from build123d import *

# Parameters (mm, degrees)
SKETCH1_W           = 10
SKETCH1_H           = 2.7
BOSS_EXTRUDE1_DEPTH = 2.7


with BuildPart() as part:
    # Sketch1 → Boss-Extrude1 (new body)
    with BuildSketch(Plane(origin=(0, 0, 0), x_dir=(0, 0, -1), z_dir=(1, 0, 0))):
        with BuildLine():
            Line((-100, -44), (-100, -60))
            Line((-100, -60), (-80, -60))
            Line((-80, -60), (-80, -50))
            Line((-80, -50), (80, -50))
            Line((80, -50), (80, -60))
            Line((80, -60), (100, -60))
            Line((100, -60), (100, -44))
            Line((100, -44), (97.3, -44))
            Line((97.3, -44), (97.3, -34))
            Line((97.3, -34), (100, -34))
            Line((100, -34), (100, -24))
            Line((100, -24), (97.3, -24))
            Line((97.3, -24), (97.3, -14))
            Line((97.3, -14), (100, -14))
            Line((100, -14), (100, -4))
            Line((100, -4), (97.3, -4))
            Line((97.3, -4), (97.3, 6))
            Line((97.3, 6), (100, 6))
            Line((100, 6), (100, 16))
            Line((100, 16), (97.3, 16))
            Line((97.3, 16), (97.3, 26))
            Line((97.3, 26), (100, 26))
            Line((100, 26), (100, 36))
            Line((100, 36), (97.3, 36))
            Line((97.3, 36), (97.3, 46))
            Line((97.3, 46), (100, 46))
            Line((100, 46), (100, 60))
            Line((100, 60), (75.851854343, 53.529523872))
            Line((75.851854343, 53.529523872), (76.550665765, 50.921524141))
            Line((76.550665765, 50.921524141), (66.891407502, 48.33333369))
            Line((66.891407502, 48.33333369), (66.19259608, 50.941333421))
            Line((66.19259608, 50.941333421), (56.533337817, 48.35314297))
            Line((56.533337817, 48.35314297), (57.232149239, 45.745143239))
            Line((57.232149239, 45.745143239), (47.572890976, 43.156952788))
            Line((47.572890976, 43.156952788), (46.874079554, 45.764952519))
            Line((46.874079554, 45.764952519), (37.214821291, 43.176762068))
            Line((37.214821291, 43.176762068), (37.913632713, 40.568762337))
            Line((37.913632713, 40.568762337), (28.25437445, 37.980571886))
            Line((28.25437445, 37.980571886), (27.555563028, 40.588571617))
            Line((27.555563028, 40.588571617), (17.896304765, 38.000381166))
            Line((17.896304765, 38.000381166), (18.595116187, 35.392381435))
            Line((18.595116187, 35.392381435), (8.935857924, 32.804190984))
            Line((8.935857924, 32.804190984), (8.237046503, 35.412190715))
            Line((8.237046503, 35.412190715), (-1.42221176, 32.824000264))
            Line((-1.42221176, 32.824000264), (-0.723400339, 30.216000533))
            Line((-0.723400339, 30.216000533), (-10.382658601, 27.627810082))
            Line((-10.382658601, 27.627810082), (-11.081470023, 30.235809813))
            Line((-11.081470023, 30.235809813), (-20.740728286, 27.647619362))
            Line((-20.740728286, 27.647619362), (-20.041916864, 25.039619631))
            Line((-20.041916864, 25.039619631), (-29.701175127, 22.45142918))
            Line((-29.701175127, 22.45142918), (-30.399986549, 25.059428911))
            Line((-30.399986549, 25.059428911), (-40.059244812, 22.47123846))
            Line((-40.059244812, 22.47123846), (-39.36043339, 19.863238729))
            Line((-39.36043339, 19.863238729), (-49.019691653, 17.275048278))
            Line((-49.019691653, 17.275048278), (-49.718503075, 19.883048009))
            Line((-49.718503075, 19.883048009), (-68.302221487, 14.903555668))
            ThreePointArc((-68.302221487, 14.903555668), (-91.366544651, -0.636913735), (-100, -27.074247963))
            Line((-100, -27.074247963), (-100, -34))
            Line((-100, -34), (-97.3, -34))
            Line((-97.3, -34), (-97.3, -44))
            Line((-97.3, -44), (-100, -44))
        make_face()
        with Locations((-82.3, -45.65)):
            Rectangle(SKETCH1_W, SKETCH1_H, mode=Mode.SUBTRACT)
        with Locations((-62.3, -45.65)):
            Rectangle(SKETCH1_W, SKETCH1_H, mode=Mode.SUBTRACT)
        with Locations((-42.3, -45.65)):
            Rectangle(SKETCH1_W, SKETCH1_H, mode=Mode.SUBTRACT)
        with Locations((-22.3, -45.65)):
            Rectangle(SKETCH1_W, SKETCH1_H, mode=Mode.SUBTRACT)
        with Locations((-2.3, -45.65)):
            Rectangle(SKETCH1_W, SKETCH1_H, mode=Mode.SUBTRACT)
        with Locations((17.7, -45.65)):
            Rectangle(SKETCH1_W, SKETCH1_H, mode=Mode.SUBTRACT)
        with Locations((37.7, -45.65)):
            Rectangle(SKETCH1_W, SKETCH1_H, mode=Mode.SUBTRACT)
        with Locations((57.7, -45.65)):
            Rectangle(SKETCH1_W, SKETCH1_H, mode=Mode.SUBTRACT)
        with Locations((77.7, -45.65)):
            Rectangle(SKETCH1_W, SKETCH1_H, mode=Mode.SUBTRACT)
    extrude(amount=BOSS_EXTRUDE1_DEPTH)


solid = part.part
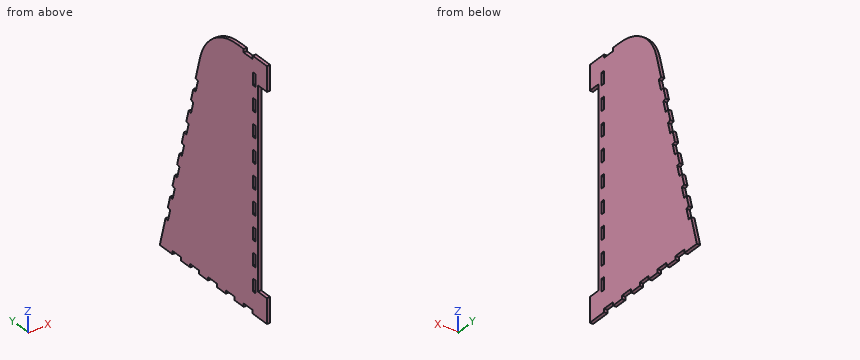
Work out the finished part from the listing and answer in its coordinate system (mm). Give positions to 0.01 mm unless a question says otherwise; leave off trailing zeros. Loops run counter-clockwise (first coordinate to the right, second up) from the corner with the lowest first, then second, coordinate; pieces in that order, holes last. Notation, with made-up numbers: (-32.75, 65.25) -> (-24.75, 65.25) arc R28 ccw to (-24.75, 103.25) -> close; hole circle Ø9 at (4, 86.5). An arc over 180 degrees is marked (long way). Use a Markdown table: item, result. Add a question column.
1. Flat-ended cylindrical pins translate along their axes: pin 1 Ø1.4 at (x, y) = (1, -45) entering from +Z; pin 2 Ø1.5 at (x, z) = (1.5, -20) entering from -Y. Find the tip coordinate at first contact, or state that the pin passes through.
2. Section A-A on y = -37.5 is taken. Determine the outline of the cut face in (x, z).
3. Find the intervals of material crossed by probe 1 along Y at (x, z) = (0.4, 43); probe 2 along Z at (x, y) = (2.4, -29); probe 3 along Y at (x, z) = (1.5, -21), in increasing order.
4. Section B-B on x = 0.7 is taken. State how many separate pieces and enclosed holes the cut face has, and give its area (3 significant figures).
5. Section C-C on z = 35 is taken. Determine the outline of the cut face in (x, y).
Results below:
| question | item | result |
|---|---|---|
| 1 | pin 1 | stops at z = 100 |
| 1 | pin 2 | stops at y = -50 |
| 2 | outline | (0, -97.3) -> (2.7, -97.3) -> (2.7, 97.3) -> (0, 97.3) -> close |
| 3 | probe 1 | y = -50 to -47, -44.3 to 18.89 |
| 3 | probe 2 | z = -100 to 100 |
| 3 | probe 3 | y = -50 to -47, -44.3 to 38.83 |
| 4 | separate pieces | 1 |
| 4 | enclosed holes | 9 |
| 4 | area | 16,200 mm^2 |
| 5 | outline | (0, -50) -> (2.7, -50) -> (2.7, 23.83) -> (0, 23.83) -> close |
